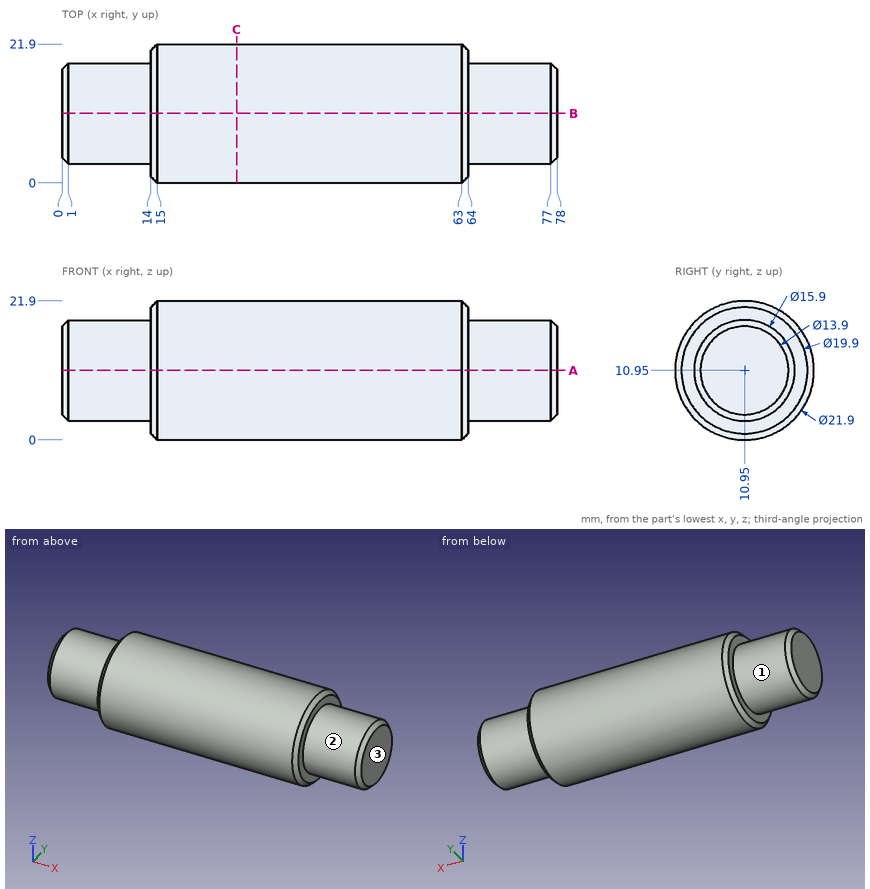
Answer from the drawing. Dimensions are ordinates in mm from the lowest x, y and z of the part. A direction names the side the tool comes from. Round coordinates to 2 decimals unless told otherwise and drop trailing zeros. Order: outer loops, then holes, each group sorted by start corner. A loop starts at its lowest first (then second) coordinate and runs counter-clockwise, first axis right, second up.
1) Flat-ended cylindrical pins translate along their axes: pin 1 (3 mm diameter, centred on y = 19.5, z = 5.5, fed in from -X); pin 2 (2 mm diameter, centred on x = 29, y = 8.5, fed in from +Z); pin 3 (3 mm diameter, centred on x = 59, z = 7, fed in from -Y). Find the tip coordinate at first contact, or state that the pin passes through.
2) Straight lines are drawn through the part: L1, parallel to X at y = 20, z = 7.25; L2, parallel to Z at x = 55.5, y = 11.5. For each, find the intervals that lie inside material, in ascending order.
3) The part is cut by section C-C on x = 27.5. Write down the section's boundary in (y, z).
4) For the marked faces 1, 2 and 3, determine the directions among +Z, -Z, +X, -X, +Y, -Y from which every point of the face is accessible in a straight line to the end or side of a thin tool.
5) The part is cut by section A-A on z = 10.95. Write down the section's boundary in (x, y).
Resolved:
1. pin 1: stops at x = 14
1. pin 2: stops at z = 21.8
1. pin 3: stops at y = 0.28
2. L1: x = 14 to 64
2. L2: z = 0.01 to 21.89
3. outline: circle Ø21.9 at (10.95, 10.95)
4. face 1: -X
4. face 2: +X
4. face 3: +Z, -Z, +X, +Y, -Y
5. outline: (0, 4) - (1, 3) - (14, 3) - (14, 1) - (15, 0) - (63, 0) - (64, 1) - (64, 3) - (77, 3) - (78, 4) - (78, 17.9) - (77, 18.9) - (64, 18.9) - (64, 20.9) - (63, 21.9) - (15, 21.9) - (14, 20.9) - (14, 18.9) - (1, 18.9) - (0, 17.9) - close
